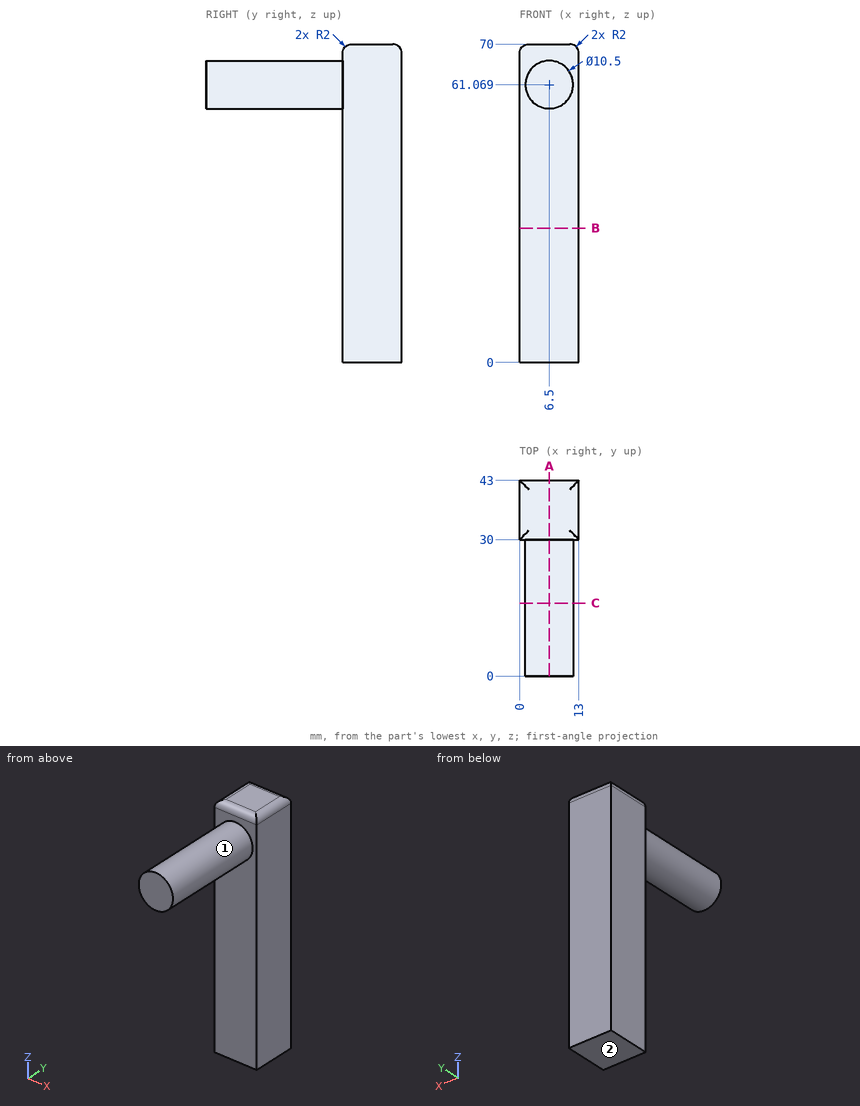
Drawing for the job (mm, zero at the part's lowest x, y, z). A direction names the side the tool comes from. Give positions to 0.01 mm unless a question says otherwise; leave off trailing zeros. Write each loop counter-clockwise with the first axis right and the second up, starting at its lowest first coordinate (ties: lowest second). Pieces come first, ordered by that corner, then holes. Notation, with made-up numbers: M 44.25,-37.5 L 98.25,-37.5 A22 cw 98.25,-25.5 Z; hole C 17.25,22.5 d4. An arc over 180 degrees is marked long. Return JSON: item names as keys, results as strings. Group by question number.
(1) Band-saw the part on C-C (y = 16). Give the cut face in (x, z), and give its area (3 significant figures).
(2) Flat gauge pins, fed straight in: pin 1 Ø4 at (x, z) = (5, 23) entering from -Y; pin 2 Ø1.5 at (y, z) = (23.5, 55.5) entering from -X (1 decimal). Where does each tip first touch, or does it go through?
(3) Band-saw the part on A-A (x = 6.5). Give the cut face in (y, z), and give its area (3 significant figures).
(4) Band-saw the part on B-B (z = 29.5). Give the cut face in (x, y).
(5) 3-axis set-ups, long thin cutter, end or side, ignore diameter. For the marked faces 1 and 2: which of +Z, -Z, +X, -X, +Y, -Y reach the whole face in a straight line?
(6) Drill centre lines: L1, parallel to Y at x = 4.5, z = 6; L2, parallel to Z at x = 6.25, y = 13 (1 decimal); L3, parallel to Z at x = 11.75, y = 35. Where is each one in solid material? Low to high. Write a range as [from, to].
Entries:
{
 "1": {"outline": "C 6.5,61.07 d10.5", "area": "86.6 mm^2"},
 "2": {"pin 1": "stops at y = 30", "pin 2": "stops at x = 4.4"},
 "3": {"outline": "M 0,55.82 L 30,55.82 L 30,0 L 43,0 L 43,68 A2 ccw 41,70 L 32,70 A2 ccw 30,68 L 30,66.32 L 0,66.32 Z", "area": "1,220 mm^2"},
 "4": {"outline": "M 0,30 L 13,30 L 13,43 L 0,43 Z"},
 "5": {"face 1": "-Y", "face 2": "-Z, +X, -X, +Y, -Y"},
 "6": {"L1": "y = [30, 43]", "L2": "z = [55.8, 66.3]", "L3": "z = [0, 69.85]"}
}
